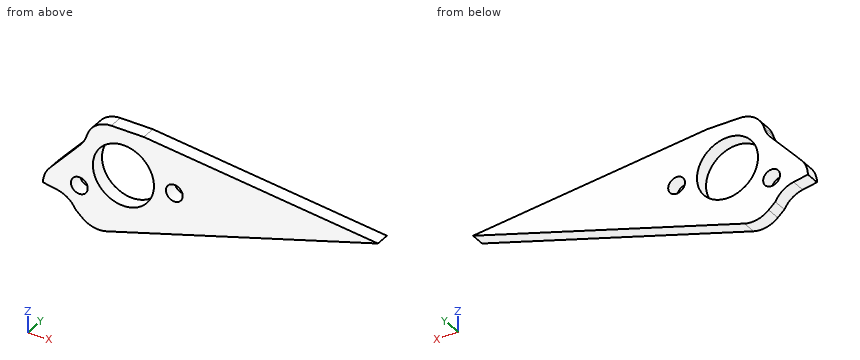
```python
from build123d import *

# Parameters (mm, degrees)
SKETCH1_R           = 6
BOSS_EXTRUDE3_DEPTH = 2.8
FILLET1_R           = 5
SKETCH5_R           = 1.65
CUT_EXTRUDE2_DEPTH  = 10
CHAMFER1_SIZE       = 6.5
CHAMFER1_SIZE_2     = 1.146125375
FILLET2_R           = 5


with BuildPart() as part:
    # Sketch1 → Boss-Extrude3 (new body)
    with BuildSketch(Plane(origin=(0, 0, 0), x_dir=(1, 0, 0), z_dir=(0, 1, 0))):
        Polygon((-9.4, 10), (-6, 13), (50, -4), (4, -9), (-6, -9), (-7.660869565, -4), (-15.8, 5), (-15.8, 8), (-9.4, 8), align=None)
        with Locations(Location((0, 0, 0), (0, 0, 270))):
            Circle(SKETCH1_R, mode=Mode.SUBTRACT)
    extrude(amount=BOSS_EXTRUDE3_DEPTH)

    # Fillet1
    fillet1_edges = [part.edges().sort_by_distance(p)[0] for p in [
        (-6, 1.4, -13),
        (-6, 1.4, 9),
        (-7.660869565, 1.4, 4),
        (-15.8, 1.4, -5),
    ]]
    fillet(fillet1_edges, radius=FILLET1_R)

    # Sketch5 → Cut-Extrude2 (cut)
    with BuildSketch(Plane.XZ):
        with Locations(Location((10, 0, 0), (0, 0, 270))):
            Circle(SKETCH5_R)
        with Locations(Location((-8.660254038, -5, 0), (0, 0, 270))):
            Circle(SKETCH5_R)
    extrude(amount=-CUT_EXTRUDE2_DEPTH, mode=Mode.SUBTRACT)

    # Chamfer1
    # the kernel refuses this chamfer: 6.5, 1.146125375 mm, written as the material it takes off along each edge
    with BuildSketch(Plane(origin=(-15.8, -16.890502177, -8), x_dir=(0.9999776716360547, 0, -0.006682531656101837), z_dir=(0, 1, 0))) as chamfer1_piece_1_section:
        Polygon((CHAMFER1_SIZE * 0.999977671636, -CHAMFER1_SIZE * 0.0066825316561), (-CHAMFER1_SIZE_2 * 0.0066825316538, -CHAMFER1_SIZE_2 * 0.999977671291), (0, 0), align=None)
    chamfer1_piece_1 = extrude(amount=36.581004353, mode=Mode.PRIVATE)
    chamfer1_piece_1 = split(chamfer1_piece_1, bisect_by=Plane(origin=(-9.4, 1.4, -7.685869002), z_dir=(-1, 0, 0)), keep=Keep.TOP, mode=Mode.PRIVATE)
    add(chamfer1_piece_1, mode=Mode.SUBTRACT)

    # Fillet2
    # the kernel refuses this fillet: 5 mm, written as the material it adds along each edge
    with BuildSketch(Plane(origin=(-9.4, 2.8, -7.982367302), x_dir=(-0.984807753012237, 0, 0.1736481776667665), z_dir=(0, -1, 0))) as fillet2_piece_1:
        with BuildLine():
            CenterArc((3.639843813, 5), FILLET2_R, 217.056619291, 52.943380709)
            Line((-0.350358241, 1.986980324), (-0.430162282, 1.92671993))
            ThreePointArc((-0.430162282, 1.92671993), (-0.273659896, 0.976125344), (-0.098480775, -0.017364818))
            Line((-0.098480775, -0.017364818), (0, -0.1))
            Line((0, -0.1), (3.639843813, -0.1))
            Line((3.639843813, -0.1), (3.639843813, 0))
        make_face()
    extrude(amount=2.8)


solid = part.part
```
Input: part model. Units: mm. Frame: model coordinates. Round coordinates to 2 decimals unless told otherwise and drop trailing zeros. Loops run counter-clockwise (first coordinate to the right, second up) from the corner with the lowest first, then second, coordinate; pieces in that order, holes last. Notation, with made-up numbers: (15, 30.25) -> (41, 30.25) arc R24 ccw to (41, 53.25) -> close; hole circle Ø2 at (-13.5, 22). An arc over 180 degrees is marked (long way). Write each question's results on one line, items separated by ' | '.
1. Section A-A (z = -5). Return loops of the section in (x, y), and give its area (3 significant figures).
Geometry results:
outline: (-15.41, 0) -> (-10.31, 0) -> (-10.31, 2.8) -> (-15.41, 2.8) -> close; (-7.01, 0) -> (-3.32, 0) -> (-3.32, 2.8) -> (-7.01, 2.8) -> close; (3.32, 0) -> (20.35, 0) -> (20.35, 2.8) -> (3.32, 2.8) -> close | area: 72.3 mm2
2. Section D-D (y = 1.6). Return loops of the section in (x, z), and give its area (3 significant figures).
Geometry results:
outline: (-15.8, -6.85) -> (-12.98, -7.35) arc R5 cw to (-9.4, -10) -> (-8.09, -11.15) arc R5 ccw to (-3.33, -12.19) -> (50, 4) -> (4, 9) -> (-2.39, 9) arc R5 ccw to (-7.14, 5.58) -> (-7.33, 5) arc R5 cw to (-8.37, 3.22) -> (-14.51, -3.57) arc R5 ccw to start; hole circle Ø3.3 at (-8.66, -5); hole circle Ø12 at (0, 0); hole circle Ø3.3 at (10, 0) | area: 602 mm2
3. Section B-B (x = 10). Return loops of the section in (y, z), and give its area (3 significant figures).
Geometry results:
outline: (0, -8.14) -> (2.8, -8.14) -> (2.8, -1.65) -> (0, -1.65) -> close; (0, 1.65) -> (2.8, 1.65) -> (2.8, 8.35) -> (0, 8.35) -> close | area: 36.9 mm2
4. Section C-C (z = -2.5). Return loops of the section in (x, y), and give its area (3 significant figures).
Geometry results:
outline: (-13.54, 0) -> (-5.45, 0) -> (-5.45, 2.8) -> (-13.54, 2.8) -> close; (5.45, 0) -> (28.59, 0) -> (28.59, 2.8) -> (5.45, 2.8) -> close | area: 87.4 mm2
5. Ray query, line 1 (Z direction, x = -9, y = 1.3); line 2 (Z direction, x = 39, y = 2.55); line 3 (Z direction, x = 21, y = 1.4). Return the intervals inside material, ascending. Write a range as from..to.
Geometry results:
line 1: -10.35..-6.61, -3.39..2.52 | line 2: 0.66..5.2 | line 3: -4.8..7.15
